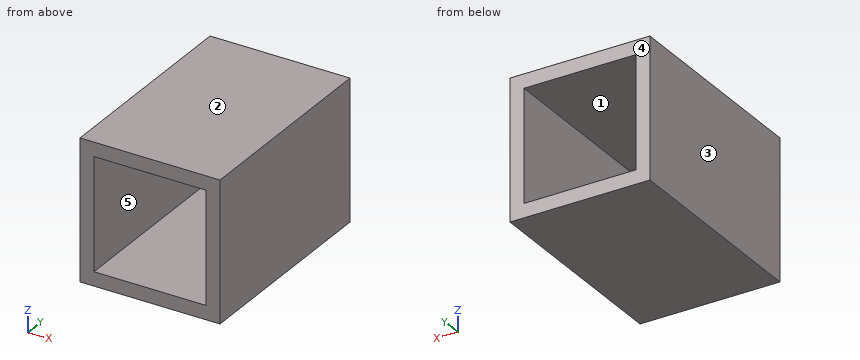
Autodesk Inventor part; units mm, degrees
ref_plane "YZ Plane" through (0, 0, 0) normal (1, 0, 0) x (0, 1, 0)
ref_plane "XZ Plane" through (0, 0, 0) normal (0, 1, 0) x (-1, 0, 0)
ref_plane "XY Plane" through (0, 0, 0) normal (0, 0, 1) x (1, 0, 0)
sketch "Sketch1" plane through (0, 0, 0) normal (1, 0, 0) x (0, 0, -1)
  line L0 (-10, -15) -> (10, -15)
  line L1 (10, -15) -> (10, 15)
  line L2 (10, 15) -> (-10, 15)
  line L3 (-10, 15) -> (-10, -15)
  line L4 (-10, -15) -> (10, 15) construction
  line L5 (10, -15) -> (-10, 15) construction
  point P0 (0, 0)
  dimension "d0" = 20
  dimension "d1" = 30
extrude "Extrusion1" add sketch "Sketch1" along normal blind 20
shell "Shell1" thickness 2 removed faces 2 at (6.6667, -15, 3.3333) at (6.6667, 15, -3.3333)
properties part number "finger_chamber"
Geometry check sheet. Reference: the model listing, model coordinates, mm. Face numbers are marked on the shaded views. A direction names the side the tool comes from. Give positions to 0.01 mm unless a question says otherwise; leave off trailing zeros. Order: outer loops, then holes, each group sorted by start corner. A loop starts at its lowest first (then second) coordinate and runs counter-clockwise, first axis right, second up. Notation, with made-up numbers: M 74,1.25 L 127,1.25 A29 cw 127,36.25 Z; hole C 75,-6 d2. An arc over 180 degrees is marked long. Use a Markdown table: item, result.
Item 1: Draft check along X on the marked faces 3, 4 and 5. Enter one of: +X half, -X half, draft (parallel to the pull), parting line (faces both ways), or undercut.
Answers follow:
| item | result |
|---|---|
| face 3 | -X half |
| face 4 | draft |
| face 5 | undercut |
Item 2: Material ranges on line 1 along Z through (x, y) = (4, -11); line 2 along X through (y, z) = (0.25, 4.5), recorded low to high.
Answers follow:
| item | result |
|---|---|
| line 1 | z = -10 to -8, 8 to 10 |
| line 2 | x = 0 to 2, 18 to 20 |
Item 3: Tool access check on the marked faces 1 and 2. Record the directions out of +Z, -Z, +X, -X, +Y, -Y that give a thin tool (end or side, any length) a straight path to the whole face; none if there is none.
Answers follow:
| item | result |
|---|---|
| face 1 | +Y, -Y |
| face 2 | +Z, +X, -X, +Y, -Y |
Item 4: Section check A-A (x = 11.25). Record the cut outline in (y, z), and give its area (3 significant figures).
Answers follow:
| item | result |
|---|---|
| outline | M -15,-10 L 15,-10 L 15,-8 L -15,-8 Z; M -15,8 L 15,8 L 15,10 L -15,10 Z |
| area | 120 mm2 |
Item 5: Section check B-B (y = 9.5). Record the cut outline in (x, z), and give its area (3 significant figures).
Answers follow:
| item | result |
|---|---|
| outline | M 0,-10 L 20,-10 L 20,10 L 0,10 Z; hole M 2,-8 L 18,-8 L 18,8 L 2,8 Z |
| area | 144 mm2 |
Item 6: Section check C-C (z = -6.25). Record the cut outline in (x, y), and give its area (3 significant figures).
Answers follow:
| item | result |
|---|---|
| outline | M 0,-15 L 2,-15 L 2,15 L 0,15 Z; M 18,-15 L 20,-15 L 20,15 L 18,15 Z |
| area | 120 mm2 |
